Verification items for the finished model (mm, model axes). Round coordinates to 2 decimals unless told otherwise and drop trailing zeros. Loops run counter-clockwise (first coordinate to the right, second up) from the corner with the lowest first, then second, coordinate; pieces in that order, holes last.
from build123d import *

# Parameters (mm, degrees)
F1_DEPTH = 56
F3_DEPTH = 56


# Not quite as in the source:
# - a feature of the source that left no trace in its solid (it failed there, or was rolled back) is left out
# - a feature names something its author has since deleted; it is built from what else it names


with BuildPart() as f1:
    # F0 (on Front) → F1 (new body)
    with BuildSketch(Plane.XZ):
        with BuildLine():
            ThreePointArc((17.0012298637, -0.0012299217), (17.0012298971, -0.0006149604), (17.0012299082, 8e-10))
            ThreePointArc((17.0012299082, 8e-10), (16.9647599435, 1.1129459753), (16.8555065268, 2.2211167615))
            Line((16.8555065268, 2.2211167615), (0.0018881159, 0.0022958043))
            Line((0.0018881159, 0.0022958043), (0.0009440615, 0.0021715172))
            Line((0.0009440615, 0.0021715172), (0.0012299082, 8e-10))
            Line((0.0012299082, 8e-10), (6.4e-09, 8e-10))
            Line((-3.33e-08, 8e-10), (-5.49e-08, -0.0012299217))
            Line((-5.49e-08, -0.0012299217), (17.0012298637, -0.0012299217))
        make_face()
        with BuildLine():
            Line((0.0018881159, 0.0022958043), (16.8555065268, 2.2211167615))
            ThreePointArc((16.8555065268, 2.2211167615), (11.2089354185, 12.7823056298), (0.0002990162, 16.9999999754))
            Line((0.0002990162, 16.9999999754), (1.31e-07, 0.0093423556))
            Line((1.31e-07, 0.0093423556), (0.0018881159, 0.0022958043))
        make_face()
        with BuildLine():
            ThreePointArc((-16.9987700918, 8e-10), (0.0006149469, -16.999999988), (17.0012298637, -0.0012299217))
            Line((17.0012298637, -0.0012299217), (-5.49e-08, -0.0012299217))
            Line((-5.49e-08, -0.0012299217), (-3.33e-08, 8e-10))
            Line((-3.33e-08, 8e-10), (2.7e-09, 0.0020472295))
            Line((2.7e-09, 0.0020472295), (1.31e-07, 0.0093423556))
            Line((1.31e-07, 0.0093423556), (-4.3972169489, 16.4211347133))
            ThreePointArc((-4.3972169489, 16.4211347133), (-13.4853114678, 10.3495507986), (-16.9987700918, 8e-10))
        make_face()
        Polygon((0.0009440615, 0.0021715172), (0.0018881159, 0.0022958043), (1.31e-07, 0.0093423556), align=None)
        Polygon((0.0009440615, 0.0021715172), (1.31e-07, 0.0093423556), (2.7e-09, 0.0020472295), align=None)
        Polygon((0.0012299082, 8e-10), (0.0009440615, 0.0021715172), (2.7e-09, 0.0020472295), (-3.33e-08, 8e-10), align=None)
    extrude(amount=F1_DEPTH)

    # F0 (on Front) → F3 (cut)
    with BuildSketch(Plane.XZ):
        with BuildLine():
            Line((1.31e-07, 0.0093423556), (0.0002990162, 16.9999999754))
            ThreePointArc((0.0002990162, 16.9999999754), (-1.1109385334, 16.9635810307), (-2.2174188682, 16.8546016754))
            Line((-2.2174188682, 16.8546016754), (1.31e-07, 0.0093423556))
        make_face()
        with BuildLine():
            Line((1.31e-07, 0.0093423556), (-2.2174188682, 16.8546016754))
            ThreePointArc((-2.2174188682, 16.8546016754), (-3.3144091037, 16.6735280601), (-4.3972169489, 16.4211347133))
            Line((-4.3972169489, 16.4211347133), (1.31e-07, 0.0093423556))
        make_face()
    extrude(amount=F3_DEPTH, mode=Mode.SUBTRACT)


solid = f1.part
1. Gauge pin test, flat ends, axial feed: P1, Ø12, axis at y = -20.5, z = -12.5, coming from the +X side; P2, Ø2, axis at x = 10.5, y = -7, coming from the +Z side; P3, Ø1.5, axis at x = -5.5, y = -8.5, coming from the +Z side. Record the tip position at first contact, or that the pin passes through.
2. Section check D-D (x = -5). Enter the section's corners in (y, z).
3. Release check for a two-part mould opening along X. For faces 1 (the face through (-2.168, -27.608, 8.1)), 2 (the face through (-0.24, 0, 0.24)) record: released by +X, released by -X, zero draft, split by the parting line, or undercut.
4. Scan lines: L1, parallel to X at y = -47, z = 8.5; L2, parallel to X at y = -46, z = 10; L3, parallel to Z at x = -6.5, y = -47.5. Record each from-to range of solid material in increasing order.
5. Section check C-C (z = 15). Enter the section's corners in (x, y), then the cut area to 3 significant figures.
6. Section check A-A (z = 11). Enter the section's corners in (x, y).
Taken from the geometry:
1. P1: stops at x = 15.71
1. P2: stops at z = 14.1
1. P3: stops at z = 16.32
2. outline: (-56, -16.25) - (0, -16.25) - (0, 16.25) - (-56, 16.25) - close
3. face 1: undercut
3. face 2: zero draft
4. L1: x = -14.72 to -2.27, 0 to 14.72
4. L2: x = -13.75 to -2.68, 0 to 13.75
4. L3: z = -15.71 to 15.71
5. outline: (-8, -56) - (-4.02, -56) - (-4.02, 0) - (-8, 0) - close; (0, -56) - (8, -56) - (8, 0) - (0, 0) - close
5. area: 671 mm2
6. outline: (-12.96, -56) - (-2.94, -56) - (-2.94, 0) - (-12.96, 0) - close; (0, -56) - (12.96, -56) - (12.96, 0) - (0, 0) - close
